Here's how the part is built. I have some questions about the finished solid (model axes, mm). A direction names the side the tool comes from. Give positions to 0.01 mm unless a question says otherwise; leave off trailing zeros. Order: outer loops, then holes, each group sorted by start corner. A loop starts at its lowest first (then second) coordinate and runs counter-clockwise, first axis right, second up.
from build123d import *

# Parameters (mm, degrees)
BOSS_EXTRUDE1_DEPTH = 1.5
SKETCH2_R           = 2.75
BOSS_EXTRUDE2_DEPTH = 6
SKETCH3_W           = 1.1
SKETCH3_H           = 1.45
SKETCH3_W_2         = 1.45
SKETCH3_H_2         = 1.1
CUT_EXTRUDE1_DEPTH  = 6
CHAMFER1_SIZE       = 0.3
FILLET1_R           = 1
FILLET3_R           = 0.2
BOSS_EXTRUDE3_DEPTH = 1
FILLET6_R           = 0.75


with BuildPart() as part:
    # Sketch1 → Boss-Extrude1 (new body)
    with BuildSketch(Plane(origin=(0, 0, 0), x_dir=(1, 0, 0), z_dir=(0, 1, 0))):
        with BuildLine():
            Line((-7.324675649, 4.396717546), (4.675324351, 4.396717546))
            ThreePointArc((4.675324351, 4.396717546), (5.382431132, 4.103824327), (5.675324351, 3.396717546))
            Line((5.675324351, 3.396717546), (5.675324351, -8.603282454))
            ThreePointArc((5.675324351, -8.603282454), (5.382431132, -9.310389235), (4.675324351, -9.603282454))
            Line((4.675324351, -9.603282454), (-7.324675649, -9.603282454))
            ThreePointArc((-7.324675649, -9.603282454), (-8.03178243, -9.310389235), (-8.324675649, -8.603282454))
            Line((-8.324675649, -8.603282454), (-8.324675649, 3.396717546))
            ThreePointArc((-8.324675649, 3.396717546), (-8.03178243, 4.103824327), (-7.324675649, 4.396717546))
        make_face()
    extrude(amount=BOSS_EXTRUDE1_DEPTH)

    # Sketch2 → Boss-Extrude2 (add)
    with BuildSketch(Plane.XZ):
        with Locations(Location((-1.324675649, 2.603282454, 0), (0, 0, 270))):
            Circle(SKETCH2_R)
    extrude(amount=BOSS_EXTRUDE2_DEPTH)

    # Sketch3 → Cut-Extrude1 (cut)
    with BuildSketch(Plane.XZ.offset(6)):
        with Locations((-1.324675649, 3.878282454)):
            Rectangle(SKETCH3_W, SKETCH3_H)
        with Locations((-0.049675649, 2.603282454)):
            Rectangle(SKETCH3_W_2, SKETCH3_H_2)
        with Locations((-1.324675649, 2.603282454)):
            Rectangle(SKETCH3_W, SKETCH3_H_2)
        with Locations((-2.599675649, 2.603282454)):
            Rectangle(SKETCH3_W_2, SKETCH3_H_2)
        with Locations((-1.324675649, 1.328282454)):
            Rectangle(SKETCH3_W, SKETCH3_H)
    extrude(amount=-CUT_EXTRUDE1_DEPTH, mode=Mode.SUBTRACT)

    # Chamfer1
    chamfer1_edges = [part.edges().sort_by_distance(p)[0] for p in [
        (-0.774675649, -6, 3.878282454),
        (-0.049675649, -6, 3.153282454),
        (0.675324351, -6, 2.603282454),
        (-0.774675649, -6, 1.328282454),
        (-2.599675649, -6, 3.153282454),
        (-1.324675649, -6, 4.603282454),
        (-1.874675649, -6, 3.878282454),
        (-3.324675649, -6, 2.603282454),
        (-2.599675649, -6, 2.053282454),
        (-1.874675649, -6, 1.328282454),
        (-1.324675649, -6, 0.603282454),
        (-0.049675649, -6, 2.053282454),
    ]]
    chamfer(chamfer1_edges, length=CHAMFER1_SIZE)

    # Fillet1
    fillet1_edges = [part.edges().sort_by_distance(p)[0] for p in [
        (-1.324675649, 0, 5.353282454),
    ]]
    fillet(fillet1_edges, radius=FILLET1_R)

    # Fillet3
    fillet3_edges = [part.edges().sort_by_distance(p)[0] for p in [
        (5.382431132, 1.5, 9.310389235),
        (-1.324675649, 0, 9.603282454),
        (-8.03178243, 0, 9.310389235),
        (5.675324351, 1.5, 2.603282454),
        (5.382431132, 1.5, -4.103824327),
        (-1.324675649, 1.5, -4.396717546),
        (-8.03178243, 1.5, -4.103824327),
        (-8.324675649, 1.5, 2.603282454),
        (-8.03178243, 1.5, 9.310389235),
        (-1.324675649, 1.5, 9.603282454),
        (-8.324675649, 0, 2.603282454),
        (-8.03178243, 0, -4.103824327),
        (-1.324675649, 0, -4.396717546),
        (5.382431132, 0, -4.103824327),
        (5.675324351, 0, 2.603282454),
        (5.382431132, 0, 9.310389235),
    ]]
    fillet(fillet3_edges, radius=FILLET3_R)

    # Sketch4 → Boss-Extrude3 (add)
    with BuildSketch(Plane(origin=(0, 1.5, 0), x_dir=(1, 0, 0), z_dir=(0, 1, 0))):
        with BuildLine():
            ThreePointArc((-0.653855256, 1.732127742), (-0.574675649, 1.396717546), (-0.653855256, 1.061307349))
            Line((-0.653855256, 1.061307349), (-1.324675649, -0.280333437))
            Line((-1.324675649, -0.280333437), (2.004503957, -6.938692651))
            ThreePointArc((2.004503957, -6.938692651), (3.010734547, -7.274102848), (3.346144744, -6.267872258))
            Line((3.346144744, -6.267872258), (-0.653855256, 1.732127742))
        make_face()
        with BuildLine():
            Line((-1.324675649, -0.280333437), (-0.653855256, 1.061307349))
            ThreePointArc((-0.653855256, 1.061307349), (-0.574675649, 1.396717546), (-0.653855256, 1.732127742))
            ThreePointArc((-0.653855256, 1.732127742), (-1.324675649, 2.146717546), (-1.995496043, 1.732127742))
            ThreePointArc((-1.995496043, 1.732127742), (-2.074675649, 1.396717546), (-1.995496043, 1.061307349))
            Line((-1.995496043, 1.061307349), (-1.324675649, -0.280333437))
        make_face()
        with BuildLine():
            Line((-4.653855256, -6.938692651), (-1.324675649, -0.280333437))
            Line((-1.324675649, -0.280333437), (-1.995496043, 1.061307349))
            ThreePointArc((-1.995496043, 1.061307349), (-2.074675649, 1.396717546), (-1.995496043, 1.732127742))
            Line((-1.995496043, 1.732127742), (-5.995496043, -6.267872258))
            ThreePointArc((-5.995496043, -6.267872258), (-5.660085846, -7.274102848), (-4.653855256, -6.938692651))
        make_face()
    extrude(amount=BOSS_EXTRUDE3_DEPTH)

    # Fillet6
    fillet6_edges = [part.edges().sort_by_distance(p)[0] for p in [
        (1.346144744, 2.5, 2.267872258),
        (-2.989265453, 2.5, 3.609513044),
        (-1.324675649, 2.5, -2.146717546),
        (-3.995496043, 2.5, 2.267872258),
        (-5.660085846, 2.5, 7.274102848),
        (0.339914154, 2.5, 3.609513044),
        (3.010734547, 2.5, 7.274102848),
    ]]
    fillet(fillet6_edges, radius=FILLET6_R - 0.0001)  # a hair under: the kernel refuses the full size


solid = part.part
Q1. For faces 1 (the face through (2, 0, 6)), 2 (the face through (-1, 1.5, 3)), 3 (the face through (0.22, 2.27, 2.9)), which set-ups out of +Z, -Z, +X, -X, +Y, -Y let a thin tool reach every point of the face, with its end or its side?
Filled sheet:
face 1: -Y
face 2: +Y
face 3: +Z, +Y
Q2. I need wall thicknesses on L1, parallel to X at y = -4.25, z = 2.5; L2, parallel to Y at x = -1.25, z = 8; L3, parallel to Z at x = -2.5, y = -4.75. Which ranges of each line are inside material? Lowest first, please.
Filled sheet:
L1: x = -4.07 to -3.32, 0.68 to 1.42
L2: y = 0 to 1.5
L3: z = 0.12 to 2.05, 3.15 to 5.09
Q3. If we section it at B-B on y = -3: List the corners of the cut face in (x, z) for me, plus the area to 3 significant figures.
Filled sheet:
outline: circle Ø5.5 at (-1.32, 2.6); hole (-3.32, 2.05) - (-1.87, 2.05) - (-1.87, 0.6) - (-0.77, 0.6) - (-0.77, 2.05) - (0.68, 2.05) - (0.68, 3.15) - (-0.77, 3.15) - (-0.77, 4.6) - (-1.87, 4.6) - (-1.87, 3.15) - (-3.32, 3.15) - close
area: 16.2 mm2
Q4. If we section it at C-C on y = -0.25: List the corners of the cut face in (x, z) for me.
Filled sheet:
outline: circle Ø6.18 at (-1.32, 2.6); hole (-3.32, 2.05) - (-1.87, 2.05) - (-1.87, 0.6) - (-0.77, 0.6) - (-0.77, 2.05) - (0.68, 2.05) - (0.68, 3.15) - (-0.77, 3.15) - (-0.77, 4.6) - (-1.87, 4.6) - (-1.87, 3.15) - (-3.32, 3.15) - close
Q5. If we section it at A-A on z = -2.75: List the corners of the cut face in (x, y) for me, plus the area to 3 significant figures.
Filled sheet:
outline: (-8.32, 0.2) arc R0.2 ccw to (-8.12, 0) - (5.48, 0) arc R0.2 ccw to (5.68, 0.2) - (5.68, 1.3) arc R0.2 ccw to (5.48, 1.5) - (-8.12, 1.5) arc R0.2 ccw to (-8.32, 1.3) - close
area: 21.0 mm2
Q6. Thinking about a two-plate mould opening in X: for faces 4 (the face through (-3.325, -3, 3)), 5 (the face through (-3.832, 2.274, 2.42)), 6 (the face through (-0.5, -3.46, -0.02)), which applies, released by +X, released by -X, zero draft, split by the parting line, or undercut?
Filled sheet:
face 4: undercut
face 5: released by -X
face 6: split by the parting line
Q7. I'm going to push flat-ended pins straight in: P1, Ø1.6, axis at x = -2, y = -2, coming from the +Z side; P2, Ø0.7, axis at y = -4, z = 4, coming from the +X side; P3, Ø1.5, axis at x = -1.5, z = 5.5, coming from the +Y side. Where does each tip first touch, or does it pass through?
Filled sheet:
P1: stops at z = 5.35
P2: stops at x = 1.22
P3: stops at y = 1.5
